Read the model definition and answer for the solid it produces. Units are mm, in the model's axes. A direction names the side the tool comes from. Coordinates: 2 decimals unless noted, no trailing zeros. Write each loop counter-clockwise with the first axis right and the second up, starting at its lowest first coordinate (ties: lowest second). Pieces come first, ordered by that corner, then holes. Notation, with made-up numbers: (47, 1.5) -> (94, 1.5) arc R10 ccw to (94, 14.5) -> close; hole circle Ø4 at (30, 45). An arc over 180 degrees is marked (long way). Use CSV: the item, a comma, the result in double quotes.
from build123d import *

# Parameters (mm, degrees)
F1_DEPTH = 55
F2_R     = 17.5
F3_DEPTH = 102
F5_DEPTH = 5
F7_DEPTH = 25
F9_DEPTH = 5
F10_SIZE = 4


with BuildPart() as f1:
    # F0 (on Top) → F1 (new body, symmetric)
    with BuildSketch(Plane.XY):
        Polygon((-13.856406, -24), (13.856406, -24), (27.712813, 0), (13.856406, 24), (-13.856406, 24), (-27.712813, 0), align=None)
    extrude(amount=F1_DEPTH, both=True)

    # F2 (on face) → F3 (cut)
    with BuildSketch(Plane.XY.offset(55)):
        Circle(F2_R)
    extrude(amount=-F3_DEPTH, mode=Mode.SUBTRACT)

    # F4 (on face) → F5 (cut)
    with BuildSketch(Plane(origin=(0, 24, 0), x_dir=(-1, 0, 0), z_dir=(0, 1, 0))):
        with BuildLine():
            ThreePointArc((0, 2), (2.12132, 2.87868), (3, 5))
            ThreePointArc((3, 5), (-2.12132, 7.12132), (0, 2))
        make_face()
    extrude(amount=-F5_DEPTH, mode=Mode.SUBTRACT)

    # F6 (on face) → F7 (cut)
    with BuildSketch(Plane.XZ.offset(24)):
        with BuildLine():
            ThreePointArc((3, -35), (2.12132, -32.87868), (0, -32))
            ThreePointArc((0, -32), (-2.12132, -37.12132), (3, -35))
        make_face()
        with BuildLine():
            ThreePointArc((0.502708, -35), (-0.355468, -35.355468), (0, -34.497292))
            ThreePointArc((0, -34.497292), (0.355468, -34.644532), (0.502708, -35))
        make_face(mode=Mode.SUBTRACT)
        with BuildLine():
            ThreePointArc((0.502708, -35), (0.355468, -34.644532), (0, -34.497292))
            ThreePointArc((0, -34.497292), (-0.355468, -35.355468), (0.502708, -35))
        make_face()
    extrude(amount=-F7_DEPTH, mode=Mode.SUBTRACT)

    # F8 (on face) → F9 (cut)
    with BuildSketch(Plane.XZ.offset(24)):
        with BuildLine():
            ThreePointArc((3, 5), (-2.12132, 7.12132), (0, 2))
            ThreePointArc((0, 2), (2.12132, 2.87868), (3, 5))
        make_face()
    extrude(amount=-F9_DEPTH, mode=Mode.SUBTRACT)

    # F10
    f10_edges = [f1.edges().sort_by_distance(p)[0] for p in [
        (-20.78461, -12, 55),
        (0, -24, 55),
        (0, 24, 55),
        (20.78461, 12, 55),
        (20.78461, -12, 55),
        (-20.78461, 12, 55),
        (-20.78461, -12, -55),
        (0, -24, -55),
        (20.78461, -12, -55),
        (20.78461, 12, -55),
        (0, 24, -55),
        (-20.78461, 12, -55),
    ]]
    chamfer(f10_edges, length=F10_SIZE)


solid = f1.part
1. Find the intervals of material crossed by line 1 along Y through (x, z) = (0, 10); line 2 along Y through (x, z) = (0, 5); line 3 along X through (y, z) = (-20.5, -35), in increasing order.
Solutions:
line 1,"y = -24 to -17.5, 17.5 to 24"
line 2,"y = -19 to -17.5, 17.5 to 19"
line 3,"x = -15.88 to -3, 3 to 15.88"
2. A tool of negligible diameter and unlimited length cuts with its end or side. For faces 5 (the flat face through (0, -22, -53)), 6 (the flat face through (0, 0, -47)), 7 (the flat face through (0, -19, 5)), 8 (the flat face through (0, 19, 5)), from which of +Z, -Z, +X, -X, +Y, -Y can it reach the whole face along a straight path? Write none if from no direction.
Solutions:
face 5,"-Z, +X, -X, -Y"
face 6,"+Z"
face 7,"-Y"
face 8,"+Y"
3. A cutting plane is placed at B-B (y = 4). Give the vertices of the cut face in (x, z), and give its area (3 significant figures).
Solutions:
outline,"(-25.4, -51) -> (-20.78, -55) -> (20.78, -55) -> (25.4, -51) -> (25.4, 51) -> (20.78, 55) -> (17.04, 55) -> (17.04, -47) -> (-17.04, -47) -> (-17.04, 55) -> (-20.78, 55) -> (-25.4, 51) -> close"
area,"2,080 mm^2"
4. Each of these flat-tipped pins is pushed along its axis until it touches: pin 1 Ø3.5 at (x, z) = (0, 5) entering from +Y; pin 2 Ø4 at (y, z) = (-19, -10.5) entering from -X; pin 3 Ø1 at (x, z) = (15, -27) entering from +Y. Where does it stop, or does it pass through?
Solutions:
pin 1,"stops at y = 19"
pin 2,"stops at x = -17.9"
pin 3,"stops at y = 22.89"
5. A cutting plane is placed at C-C (x = -20.5). Give the vertices of the cut face in (y, z).
Solutions:
outline,"(-12.49, -51) -> (-4.49, -55) -> (4.49, -55) -> (12.49, -51) -> (12.49, 51) -> (4.49, 55) -> (-4.49, 55) -> (-12.49, 51) -> close"
6. A cutting plane is placed at A-A (z = -45.5). Give the vertices of the cut face in (x, y).
Solutions:
outline,"(-27.71, 0) -> (-13.86, -24) -> (13.86, -24) -> (27.71, 0) -> (13.86, 24) -> (-13.86, 24) -> close; hole circle Ø35 at (0, 0)"
7. A cutting plane is placed at D-D (x = 9.5). Give the vertices of the cut face in (y, z).
Solutions:
outline,"(-24, -51) -> (-20, -55) -> (20, -55) -> (24, -51) -> (24, 51) -> (20, 55) -> (14.7, 55) -> (14.7, -47) -> (-14.7, -47) -> (-14.7, 55) -> (-20, 55) -> (-24, 51) -> close"
8. For a pull along Y with two mould halves and no side action, classify faces 1 (the flat face through (17, 5, 55)), 2 (the flat face through (-20.688, 12.168, 0.714)), 3 (the flat face through (0, -22, 53)), 4 (the cylindrical face through (-13.887, -10.648, 4.714)) as pulls with the +Y half, pulls with the -Y half, needs draft (parallel to the pull), parting line crosses it, or undercut.
Solutions:
face 1,"needs draft"
face 2,"pulls with the +Y half"
face 3,"pulls with the -Y half"
face 4,"undercut"
